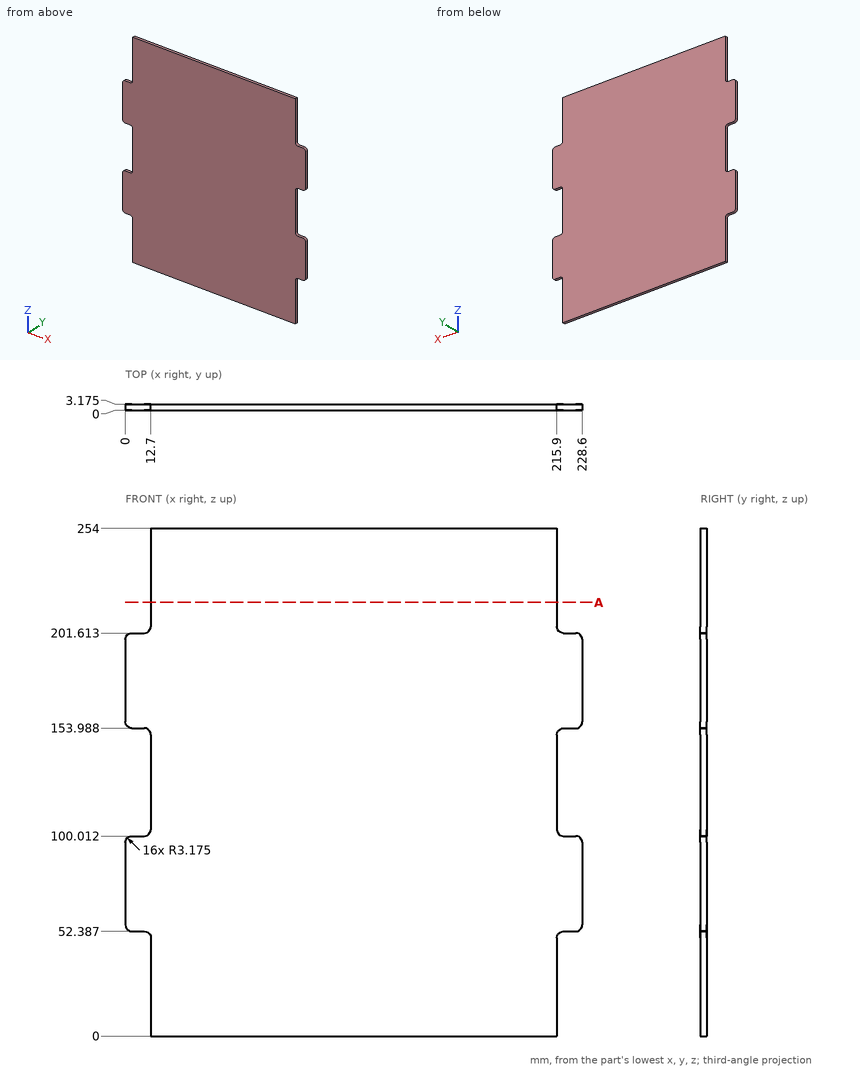
Geometry check sheet. Reference: drawing and pictorial views, mm from the part's lowest x, y, z. Give positions to 0.01 mm unless a question says otherwise; leave off trailing zeros. Order: outer loops, then holes, each group sorted by start corner. A loop starts at its lowest first (then second) coordinate and runs counter-clockwise, first axis right, second up. Notation, with made-up numbers: (41.25, 47) - (60.25, 47) arc R28 cw to (60.25, 85) - close; hole circle Ø2 at (-22.5, 72.5). An arc over 180 degrees is marked (long way). Use one line per item in the form item = value.
1) Material ranges on probe 1 along X at (y, z) = (1.45, 14); probe 2 along X at (y, z) = (1.2, 53), recorded low to high. Write a range as from..to.
Working result:
probe_1 = 12.7..215.9
probe_2 = 1.3..227.3
2) Sectioned sample at A-A (z = 217). Record the boundary of the cut face in (x, y) (1 decimal).
Working result:
outline = (12.7, 0) - (215.9, 0) - (215.9, 3.2) - (12.7, 3.2) - close
3) Depth check by flat-ended pin: pin 1 Ø1 at (x, y) = (5, 1.5) entering from +Z; pin 2 Ø1 at (y, z) = (2, 20) entering from +X; pin 3 Ø1.6 at (y, z) = (2, 16) entering from -X. Enter the tip coordinate at first touch or a pass-through.
Working result:
pin_1 = 201.61
pin_2 = 215.9
pin_3 = 12.7
